```python
from build123d import *

# Parameters (mm, degrees)
SKETCH1_W                 = 50.8
SKETCH1_H                 = 127
BOSS_EXTRUDE1_DEPTH       = 9.525
SKETCH2_W                 = 50.8
SKETCH2_H                 = 152.4
CUT_EXTRUDE1_DEPTH        = 70.051688068
F_8_CLEARANCE_HOLE1_D     = 4.4958
F_8_CLEARANCE_HOLE2_D     = 4.4958
F_8_CLEARANCE_HOLE2_DEPTH = 13.97
F_8_CLEARANCE_HOLE2_TIP   = 1.350674586
F_8_CLEARANCE_HOLE3_D     = 4.4958
F_8_CLEARANCE_HOLE3_DEPTH = 13.97
F_8_CLEARANCE_HOLE3_TIP   = 1.350674586
SKETCH12_W                = 6.35
SKETCH12_H                = 7.62
CUT_EXTRUDE2_DEPTH        = 70.051688068


with BuildPart() as part:
    # Sketch1 → Boss-Extrude1 (new body)
    with BuildSketch(Plane(origin=(0, 0, 0), x_dir=(1, 0, 0), z_dir=(0, 1, 0))):
        Rectangle(SKETCH1_W, SKETCH1_H)
    extrude(amount=BOSS_EXTRUDE1_DEPTH)

    # Sketch2 → Cut-Extrude1 (cut, through all)
    with BuildSketch(Plane(origin=(0, 9.525, 0), x_dir=(1, 0, 0), z_dir=(0, 1, 0))):
        with Locations((0, -25.4)):
            Rectangle(SKETCH2_W, SKETCH2_H)
    extrude(amount=-CUT_EXTRUDE1_DEPTH, mode=Mode.SUBTRACT)

    # #8 Clearance Hole1 (through all)
    with Locations(Plane(origin=(0, 9.525, 0), x_dir=(1, 0, 0), z_dir=(0, 1, 0))):
        with Locations((0, 57.15)):
            Hole(F_8_CLEARANCE_HOLE1_D / 2)

    # #8 Clearance Hole2
    with Locations(Plane.ZY.offset(25.4)):
        with Locations((-57.15, 4.7625)):
            Hole(F_8_CLEARANCE_HOLE2_D / 2, depth=F_8_CLEARANCE_HOLE2_DEPTH)
            with Locations((0, 0, -(F_8_CLEARANCE_HOLE2_DEPTH + F_8_CLEARANCE_HOLE2_TIP / 2))):  # 118° drill point
                Cone(0, F_8_CLEARANCE_HOLE2_D / 2, F_8_CLEARANCE_HOLE2_TIP, mode=Mode.SUBTRACT)

    # #8 Clearance Hole3
    with Locations(Plane(origin=(25.4, 0, 0), x_dir=(0, 0, -1), z_dir=(1, 0, 0))):
        with Locations((57.15, 4.7625)):
            Hole(F_8_CLEARANCE_HOLE3_D / 2, depth=F_8_CLEARANCE_HOLE3_DEPTH)
            with Locations((0, 0, -(F_8_CLEARANCE_HOLE3_DEPTH + F_8_CLEARANCE_HOLE3_TIP / 2))):  # 118° drill point
                Cone(0, F_8_CLEARANCE_HOLE3_D / 2, F_8_CLEARANCE_HOLE3_TIP, mode=Mode.SUBTRACT)

    # Sketch12 → Cut-Extrude2 (cut, through all)
    with BuildSketch(Plane(origin=(0, 9.525, 0), x_dir=(1, 0, 0), z_dir=(0, 1, 0))):
        with Locations((-18.415, 57.15)):
            Rectangle(SKETCH12_W, SKETCH12_H)
        with Locations((18.415, 57.15)):
            Rectangle(SKETCH12_W, SKETCH12_H)
    extrude(amount=-CUT_EXTRUDE2_DEPTH, mode=Mode.SUBTRACT)


solid = part.part
```
Part model, mm, in its own coordinate system. A direction names the side the tool comes from. Round coordinates to 2 decimals unless told otherwise and drop trailing zeros. Order: outer loops, then holes, each group sorted by start corner. A loop starts at its lowest first (then second) coordinate and runs counter-clockwise, first axis right, second up. Notation, with made-up numbers: M -6,16 L 44,16 A21 cw 44,55 Z; hole C 21.5,16.25 d2. An arc over 180 degrees is marked long. Answer in a Markdown table with one row per item. Add a question column.
Q1. Cut at A-A on x = 0. Give the cut face in (y, z) (3 decimals).
Q2. Wall check: L1, parallel to X at y = 7.5, z = -54.25; L2, parallel to Z at x = -17, y = 9.25; L3, parallel to Y at x = -12.4, z = -57.15 (3 decimals). Give the ranges that are in metal, low to high. Write a range as from..to.
Q3. Mould opens along X. For faces 5 (the face through (-15.24, 7, -56)), 6 (the face through (0, 9.525, -60)), 7 (the face through (-10.314, 4.88, -56.778)) say: +X half, -X half, draft (parallel to the pull), parting line (faces both ways), or undercut.
Q4. Cut at C-C on x = -16. Give the cut face in (y, z) (3 decimals), and give its area (3 significant figures).
Q5. Pin check, flat tips, straight feed: pin 1 (5 mm diameter, centred on y = 4.76, z = -57.15, fed in from -X); pin 2 (2.5 mm diameter, centred on y = 4.5, z = -58, fed in from -X); pin 3 (2.5 mm diameter, centred on y = 4.76, z = -57.15, fed in from +X); pin 4 (3.5 mm diameter, centred on y = 4.76, z = -57.15, fed in from -X). Stop position of each tip, or through.
Q6. 3-axis set-ups, long thin cutter, end or side, ignore diameter. For faces 1 (the face through (-13.31, 3.39, -55.37)), 2 (the face through (23.47, 3.39, -58.93)), 3 (the face through (0, 5, -50.8)), 4 (the face through (-18, 5, -53.34)): which of +Z, -Z, +X, -X, +Y, -Y reach the whole face in a straight line?
Q7. Cut at B-B on z = -56.5. Give the number of separate pieces and of enclosed holes in the cut face, and give its area (3 significant figures).
Established:
| question | item | result |
|---|---|---|
| 1 | outline | M 0,-63.5 L 9.525,-63.5 L 9.525,-59.398 L 0,-59.398 Z; M 0,-54.902 L 9.525,-54.902 L 9.525,-50.8 L 0,-50.8 Z |
| 2 | L1 | x = -25.4..-21.59, -15.24..15.24, 21.59..25.4 |
| 2 | L2 | z = -63.5..-60.96, -53.34..-50.8 |
| 2 | L3 | y = 0..2.515, 7.01..9.525 |
| 3 | face 5 | undercut |
| 3 | face 6 | draft |
| 3 | face 7 | -X half |
| 4 | outline | M 0,-63.5 L 9.525,-63.5 L 9.525,-60.96 L 0,-60.96 Z; M 0,-53.34 L 9.525,-53.34 L 9.525,-50.8 L 0,-50.8 Z |
| 4 | area | 48.4 mm2 |
| 5 | pin 1 | stops at x = -25.4 |
| 5 | pin 2 | stops at x = -11.36 |
| 5 | pin 3 | stops at x = 10.83 |
| 5 | pin 4 | stops at x = -11.13 |
| 6 | face 1 | -X |
| 6 | face 2 | +X |
| 6 | face 3 | +Z, +X, -X, +Y, -Y |
| 6 | face 4 | +Y, -Y |
| 7 | separate pieces | 6 |
| 7 | enclosed holes | 0 |
| 7 | area | 251 mm2 |
